CAD build for the part. Positions are in the model's coordinates, mm. Face numbers are marked on the shaded views. A direction names the side the tool comes from. Round coordinates to 2 decimals unless told otherwise and drop trailing zeros. Loops run counter-clockwise (first coordinate to the right, second up) from the corner with the lowest first, then second, coordinate; pieces in that order, holes last.
```python
from build123d import *

# Parameters (mm, degrees)
SKETCH1_W           = 90
SKETCH1_H           = 60
BOSS_EXTRUDE1_DEPTH = 30
SKETCH2_W           = 40.3
SKETCH2_H           = 40
CUT_EXTRUDE1_DEPTH  = 61
SKETCH3_R           = 4.1
CUT_EXTRUDE2_DEPTH  = 31
SKETCH4_R           = 8.8
CUT_EXTRUDE3_DEPTH  = 10
CHAMFER1_SIZE       = 1


with BuildPart() as part:
    # Sketch1 → Boss-Extrude1 (new body)
    with BuildSketch(Plane(origin=(0, 0, 0), x_dir=(1, 0, 0), z_dir=(0, 1, 0))):
        Rectangle(SKETCH1_W, SKETCH1_H)
    extrude(amount=BOSS_EXTRUDE1_DEPTH)

    # Sketch2 → Cut-Extrude1 (cut, through all)
    with BuildSketch(Plane.XY.offset(30)):
        with Locations((0, 30)):
            Rectangle(SKETCH2_W, SKETCH2_H)
    extrude(amount=-CUT_EXTRUDE1_DEPTH, mode=Mode.SUBTRACT)

    # Sketch3 → Cut-Extrude2 (cut, through all)
    with BuildSketch(Plane.XZ):
        with Locations((-35, 15)):
            Circle(SKETCH3_R)
        with Locations((-35, -15)):
            Circle(SKETCH3_R)
        with Locations((35, -14.217273236)):
            Circle(SKETCH3_R)
        with Locations((35, 15)):
            Circle(SKETCH3_R)
    extrude(amount=-CUT_EXTRUDE2_DEPTH, mode=Mode.SUBTRACT)

    # Sketch4 → Cut-Extrude3 (cut)
    with BuildSketch(Plane.XZ):
        with Locations((35, 15)):
            Circle(SKETCH4_R)
        with Locations((35, -14.217273236)):
            Circle(SKETCH4_R)
        with Locations((-35, 15)):
            Circle(SKETCH4_R)
        with Locations((-35, -15)):
            Circle(SKETCH4_R)
    extrude(amount=-CUT_EXTRUDE3_DEPTH, mode=Mode.SUBTRACT)

    # Chamfer1
    chamfer1_edges = [part.edges().sort_by_distance(p)[0] for p in [
        (20.15, 30, 0),
        (-20.15, 30, 0),
    ]]
    chamfer(chamfer1_edges, length=CHAMFER1_SIZE)


solid = part.part
```
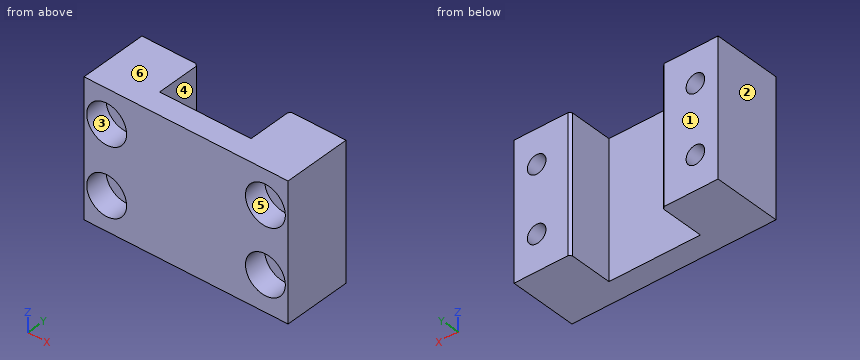
Item 1: 3-axis set-ups, long thin cutter, end or side, ignore diameter. For the marked faces 4, 5 and 6: which of +Z, -Z, +X, -X, +Y, -Y reach the whole face in a straight line?
Answers follow:
face 4: +Z, -Z, +Y
face 5: -Y
face 6: +Z, +X, -X, +Y, -Y
Item 2: Cut at B-B, the plane z = 15. Give the cut face in (x, y), plus the area to 3 significant figures.
Answers follow:
outline: (-45, 0) - (-43.8, 0) - (-43.8, 10) - (-39.1, 10) - (-39.1, 30) - (-45, 30) - close; (-30.9, 10) - (-26.2, 10) - (-26.2, 0) - (26.2, 0) - (26.2, 10) - (30.9, 10) - (30.9, 30) - (21.15, 30) - (20.15, 29) - (20.15, 10) - (-20.15, 10) - (-20.15, 29) - (-21.15, 30) - (-30.9, 30) - close; (39.1, 10) - (43.8, 10) - (43.8, 0) - (45, 0) - (45, 30) - (39.1, 30) - close
area: 1,210 mm2
Item 3: Cut at A-A, the plane y = 14.5. Give the cut face in (x, z).
Answers follow:
outline: (-45, -30) - (-20.15, -30) - (-20.15, 30) - (-45, 30) - close; (20.15, -30) - (45, -30) - (45, 30) - (20.15, 30) - close; hole circle Ø8.2 at (-35, -15); hole circle Ø8.2 at (-35, 15); hole circle Ø8.2 at (35, -14.22); hole circle Ø8.2 at (35, 15)
Item 4: Two-plate mould, pull along X, no slides. Class the marked faces 1, 2 and 3: released by +X, released by -X, zero draft, split by the parting line, or undercut.
Answers follow:
face 1: zero draft
face 2: released by -X
face 3: undercut
Item 5: Probe line 1 (Z direction, x = -35, y = 5); line 2 (X direction, y = 19.5, z = -4.5); line 3 (Z direction, x = 35, y = 2). List the from-to ranges inside material, lowest first.
Answers follow:
line 1: z = -30 to -23.8, -6.2 to 6.2, 23.8 to 30
line 2: x = -45 to -20.15, 20.15 to 45
line 3: z = -30 to -23.02, -5.42 to 6.2, 23.8 to 30
Item 6: Cut at D-D, the plane y = 9. Give the cut face in (x, z), plus the area to 3 significant figures.
Answers follow:
outline: (-45, -30) - (45, -30) - (45, 30) - (-45, 30) - close; hole circle Ø17.6 at (-35, -15); hole circle Ø17.6 at (-35, 15); hole circle Ø17.6 at (35, -14.22); hole circle Ø17.6 at (35, 15)
area: 4,430 mm2
Item 7: Flat gauge pins, fed straight in: P1, Ø10.5, axis at x = -35, z = 15, coming from the -Y side; P2, Ø5, axis at x = -35, z = 15, coming from the -Y side. Where does each tip first touch, or does it go through?
Answers follow:
P1: stops at y = 10
P2: passes through
Item 8: Cut at C-C, the plane x = 35. Give the cut face in (y, z), plus the area to 3 significant figures.
Answers follow:
outline: (0, -30) - (30, -30) - (30, -18.32) - (10, -18.32) - (10, -23.02) - (0, -23.02) - close; (0, -5.42) - (10, -5.42) - (10, -10.12) - (30, -10.12) - (30, 10.9) - (10, 10.9) - (10, 6.2) - (0, 6.2) - close; (0, 23.8) - (10, 23.8) - (10, 19.1) - (30, 19.1) - (30, 30) - (0, 30) - close
area: 1,120 mm2
